Geometry: final body of the model. Coordinates: model frame, mm. A direction names the side the tool comes from. Coordinates: 2 decimals unless noted, no trailing zeros. Loops run counter-clockwise (first coordinate to the right, second up) from the corner with the lowest first, then second, coordinate; pieces in that order, holes last. Notation, with made-up numbers: (33, 57.25) - (60, 57.25) arc R21 cw to (60, 76.25) - close; hole circle Ø10 at (-17, 65.5). An arc over 180 degrees is marked (long way). Return JSON: item names as keys, results as strings.
from build123d import *

# Parameters (mm, degrees)
SKETCH1_W           = 120
SKETCH1_H           = 85
BOSS_EXTRUDE1_DEPTH = 5
SKETCH2_W           = 5
SKETCH2_H           = 10
BOSS_EXTRUDE2_DEPTH = 15
SKETCH3_R           = 2.5
CUT_EXTRUDE1_DEPTH  = 129.865239689
SKETCH5_W           = 5
SKETCH5_H           = 25
SKETCH5_H_2         = 15
CUT_EXTRUDE2_DEPTH  = 76.041655099
CHAMFER1_SIZE       = 5
SKETCH6_W           = 110
SKETCH6_H           = 10
CUT_EXTRUDE3_DEPTH  = 77.198753271


with BuildPart() as part:
    # Sketch1 → Boss-Extrude1 (new body)
    with BuildSketch(Plane(origin=(0, 0, 0), x_dir=(1, 0, 0), z_dir=(0, 1, 0))):
        Rectangle(SKETCH1_W, SKETCH1_H)
    extrude(amount=BOSS_EXTRUDE1_DEPTH)

    # Sketch2 → Boss-Extrude2 (add)
    with BuildSketch(Plane(origin=(0, 5, 0), x_dir=(1, 0, 0), z_dir=(0, 1, 0))):
        with Locations((-57.5, 12.5)):
            Rectangle(SKETCH2_W, SKETCH2_H)
        with Locations((-57.5, -12.5)):
            Rectangle(SKETCH2_W, SKETCH2_H)
        with Locations((57.5, -12.5)):
            Rectangle(SKETCH2_W, SKETCH2_H)
        with Locations((57.5, 12.5)):
            Rectangle(SKETCH2_W, SKETCH2_H)
    extrude(amount=BOSS_EXTRUDE2_DEPTH)

    # Sketch3 → Cut-Extrude1 (cut, through all)
    with BuildSketch(Plane.ZY.offset(60)):
        with Locations((-12.5, 15)):
            Circle(SKETCH3_R)
        with Locations((12.5, 15)):
            Circle(SKETCH3_R)
    extrude(amount=-CUT_EXTRUDE1_DEPTH, mode=Mode.SUBTRACT)

    # Sketch5 → Cut-Extrude2 (cut, through all)
    with BuildSketch(Plane(origin=(0, 5, 0), x_dir=(1, 0, 0), z_dir=(0, 1, 0))):
        with Locations((-57.5, 30)):
            Rectangle(SKETCH5_W, SKETCH5_H)
        with Locations((-57.5, 0)):
            Rectangle(SKETCH5_W, SKETCH5_H_2)
        with Locations((-57.5, -30)):
            Rectangle(SKETCH5_W, SKETCH5_H)
        with Locations((57.5, -30)):
            Rectangle(SKETCH5_W, SKETCH5_H)
        with Locations((57.5, 0)):
            Rectangle(SKETCH5_W, SKETCH5_H_2)
        with Locations((57.5, 30)):
            Rectangle(SKETCH5_W, SKETCH5_H)
    extrude(amount=-CUT_EXTRUDE2_DEPTH, mode=Mode.SUBTRACT)

    # Chamfer1
    chamfer1_edges = [part.edges().sort_by_distance(p)[0] for p in [
        (-60, 0, 12.5),
        (-60, 0, -12.5),
        (60, 0, -12.5),
        (60, 0, 12.5),
    ]]
    chamfer(chamfer1_edges, length=CHAMFER1_SIZE)

    # Sketch6 → Cut-Extrude3 (cut, through all)
    with BuildSketch(Plane.XZ):
        Polygon((-55, -7.5), (55, -7.5), (55, -17.5), (55, -42.5), (-55, -42.5), (-55, -17.5), align=None)
        Polygon((-60, -7.5), (-60, -42.5), (-55, -42.5), (-55, -17.5), (-55, -7.5), align=None)
        with Locations((0, 37.5)):
            Rectangle(SKETCH6_W, SKETCH6_H)
        Polygon((55, -42.5), (60, -42.5), (60, -7.5), (55, -7.5), (55, -17.5), align=None)
    extrude(amount=-CUT_EXTRUDE3_DEPTH, mode=Mode.SUBTRACT)


solid = part.part
Item 1: Reachability of faces 5 (the face through (-55, 3, 25)), 6 (the face through (-55, 3, 0)), 7 (the face through (55, 12, 13)), 8 (the face through (55, 3, 25)), 9 (the face through (55, 3, 0)) from +Z, -Z, +X, -X, +Y, -Y: full face, straight path, thin tool, end or side. Return the list, or none.
Worked out:
{"face 5": "+Z, -X, +Y, -Y", "face 6": "-Z, -X, +Y, -Y", "face 7": "+Z, -Z, +Y", "face 8": "+Z, +X, +Y, -Y", "face 9": "-Z, +X, +Y, -Y"}
Item 2: First-contact query: pin 1 Ø1.5 at (y, z) = (3, 26) entering from -X; pin 2 Ø3 at (y, z) = (15.5, 12) entering from -X; pin 3 Ø8 at (y, z) = (15, 12.5) entering from -X; pin 4 Ø2.5 at (x, y) = (56.5, 7.5) entering from -Z. Flat tips, straight axial feed; report the tip coordinate or a pass-through.
Worked out:
{"pin 1": "x = -55", "pin 2": "through", "pin 3": "x = -60", "pin 4": "z = 7.5"}
Item 3: Section query C-C, the plane y = 3.5. Return loops of the section in (x, z).
Worked out:
{"outline": "(-58.5, 7.5) - (-55, 7.5) - (-55, -7.5) - (55, -7.5) - (55, 7.5) - (58.5, 7.5) - (58.5, 17.5) - (55, 17.5) - (55, 32.5) - (-55, 32.5) - (-55, 17.5) - (-58.5, 17.5) - close"}
Item 4: Mould query, pull axis Y, two halves, no side actions, for faces 1 (the face through (57, 12, 17.5)), 2 (the face through (57, 15, 10)), 3 (the face through (-58, 15, 10)), 4 (the face through (-1, 0, 12)). Classes: +Y half, -Y half, draft (parallel to the pull), parting line (faces both ways), or undercut.
Worked out:
{"face 1": "draft", "face 2": "undercut", "face 3": "undercut", "face 4": "-Y half"}
Item 5: Ray query, probe 1 along X at (y, z) = (13.5, 17); probe 2 along X at (y, z) = (1.5, -1); probe 3 along Y at (x, z) = (12, 21). Return the intervals inside material, ascending. Write a range as from..to.
Worked out:
{"probe 1": "-60..-55, 55..60", "probe 2": "-55..55", "probe 3": "0..5"}
Item 6: Section query D-D, the plane x = -48. Return loops of the section in (y, z), and give its area (3 significant figures).
Worked out:
{"outline": "(0, -7.5) - (5, -7.5) - (5, 32.5) - (0, 32.5) - close", "area": "200 mm^2"}
Item 7: Section query B-B, the plane z = 12.5. Return loops of the section in (x, y).
Worked out:
{"outline": "(-60, 5) - (-55, 0) - (55, 0) - (60, 5) - (60, 12.5) - (55, 12.5) - (55, 5) - (-55, 5) - (-55, 12.5) - (-60, 12.5) - close; (-60, 17.5) - (-55, 17.5) - (-55, 20) - (-60, 20) - close; (55, 17.5) - (60, 17.5) - (60, 20) - (55, 20) - close"}
Item 8: Section query A-A, the plane y = 8.5. Return loops of the section in (x, z).
Worked out:
{"outline": "(-60, 7.5) - (-55, 7.5) - (-55, 17.5) - (-60, 17.5) - close; (55, 7.5) - (60, 7.5) - (60, 17.5) - (55, 17.5) - close"}
